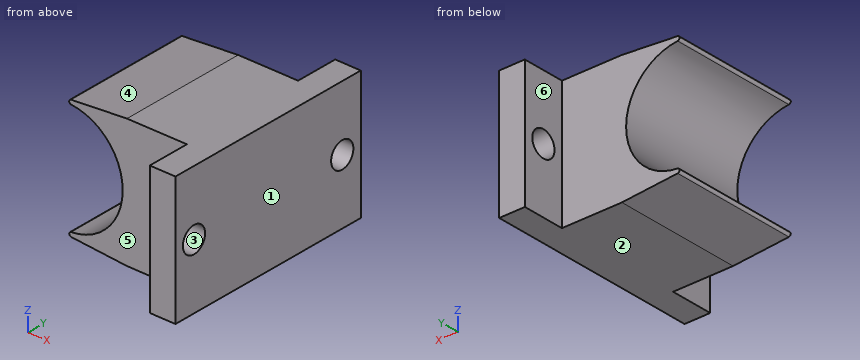
```python
from build123d import *

# Parameters (mm, degrees)
SKETCH003_W     = 5
SKETCH003_H     = 25
SKETCH003_R     = 1.5
PAD001_DEPTH    = 10
SKETCH004_W     = 5
SKETCH004_H     = 5
POCKET002_DEPTH = 7
PAD009_DEPTH    = 5
PAD010_DEPTH    = 5
PAD011_DEPTH    = 15


with BuildPart() as part:
    # Sketch003 (on DatumPlane) → Pad001 (new body)
    with BuildSketch(Plane(origin=(0, 0, 0), x_dir=(0, 0, -1), z_dir=(-1, 0, 0))):
        with Locations((-10, 20)):
            Rectangle(SKETCH003_W, SKETCH003_H)
        with Locations((-10, 30)):
            Circle(SKETCH003_R, mode=Mode.SUBTRACT)
        with Locations((-10, 10)):
            Circle(SKETCH003_R, mode=Mode.SUBTRACT)
    extrude(amount=PAD001_DEPTH)

    # Sketch004 (on Face8 of Pad001) → Pocket002 (cut)
    with BuildSketch(Plane(origin=(-10, 0, 0), x_dir=(0, 0, -1), z_dir=(-1, 0, 0))):
        with Locations((-10, 30)):
            Rectangle(SKETCH004_W, SKETCH004_H)
        with Locations((-10, 10)):
            Rectangle(SKETCH004_W, SKETCH004_H)
    extrude(amount=-POCKET002_DEPTH, mode=Mode.SUBTRACT)

    # Pocket002 Face3 → Pad009 (add)
    with BuildSketch(Plane(origin=(-4.416667, -20, 7.5), x_dir=(0, -1, 0), z_dir=(0, 0, -1))):
        Polygon((-12.5, -4.416667), (12.5, -4.416667), (12.5, -1.416667), (7.5, -1.416667), (7.5, 5.583333), (-7.5, 5.583333), (-7.5, -1.416667), (-12.5, -1.416667), align=None)
    extrude(amount=PAD009_DEPTH)

    # Pad009 Face3 → Pad010 (add)
    with BuildSketch(Plane(origin=(-4.416667, -20, 12.5), x_dir=(0, 1, 0), z_dir=(0, 0, 1))):
        Polygon((-12.5, -4.416667), (12.5, -4.416667), (12.5, -1.416667), (7.5, -1.416667), (7.5, 5.583333), (-7.5, 5.583333), (-7.5, -1.416667), (-12.5, -1.416667), align=None)
    extrude(amount=PAD010_DEPTH)

    # Sketch020 (on Face11 of Pad010) → Pad011 (join)
    with BuildSketch(Plane(origin=(0, -12.5, 0), x_dir=(0, 0, -1), z_dir=(0, 1, 0))):
        with BuildLine():
            ThreePointArc((-16.482143, 16.518519), (-10, 10.5), (-3.517857, 16.518519))
            ThreePointArc((-3.019333, 16.519851), (-3.269212, 16.749999), (-3.517857, 16.518519))
            Line((-2.5, 10), (-3.019333, 16.519851))
            Line((-2.5, 10), (-10, 10))
            Line((-17.5, 10), (-10, 10))
            Line((-17.5, 10), (-16.980667, 16.519851))
            ThreePointArc((-16.482143, 16.518519), (-16.730788, 16.749999), (-16.980667, 16.519851))
        make_face()
    extrude(amount=-PAD011_DEPTH)


solid = part.part
```
Check sheet for the modelled part. Datum: model origin and axes. Units: mm. Face numbers are marked on the shaded views. A direction names the side the tool comes from. Round coordinates to 2 decimals unless told otherwise and drop trailing zeros. Order: outer loops, then holes, each group sorted by start corner. A loop starts at its lowest first (then second) coordinate and runs counter-clockwise, first axis right, second up. Notation, with made-up numbers: (-17, 37.25) - (8, 37.25) arc R8 ccw to (8, 43.25) - close; hole circle Ø3 at (12, 37.25). An arc over 180 degrees is marked (long way). Write item = value, one per line.
Q1. Thickness scan on line 1 along Y through (x, z) = (-1.35, 10); line 2 along Z through (x, y) = (-0.85, -30); line 3 along X through (y, z) = (-11.5, 14.75). Record the ranges inside material, lowest first.
Computed:
line_1 = -32.5 to -31.5, -28.5 to -11.5, -8.5 to -7.5
line_2 = 2.5 to 8.5, 11.5 to 17.5
line_3 = -3 to 0
Q2. Go/stop test with flat-tipped pins: pin 1 (4 mm diameter, centred on x = -13.5, y = -12, fed in from +Z); pin 2 (6 mm diameter, centred on x = -12.5, z = 7, fed in from -Y); pin 3 (1.5 mm diameter, centred on y = -29, z = 8.5, fed in from -X). Record where each tip stops, or that it passes through.
Computed:
pin_1 = 17.38
pin_2 = -27.5
pin_3 = -3
Q3. Section check C-C (y = -10). Record the boundary of the cut face in (x, z), and give its area (3 significant figures).
Computed:
outline = (-3, 2.5) - (0, 2.5) - (0, 8.5) - (-3, 8.5) - close; (-3, 11.5) - (0, 11.5) - (0, 17.5) - (-3, 17.5) - close
area = 36.0 mm^2
Q4. Tool access check on the marked faces 4, 5 and 6. Record the directions out of +Z, -Z, +X, -X, +Y, -Y that give a thin tool (end or side, any length) a straight path to the whole face; none if there is none.
Computed:
face_4 = +Z, -X, +Y, -Y
face_5 = +Z, -Z, -X, -Y
face_6 = +Z, -Z, -X, +Y
Q5. Draft check along Z on the marked faces 1, 2 and 3. Enter one of: pulls with the +Z half, pulls with the -Z half, needs draft (parallel to the pull), parting line crosses it, or undercut.
Computed:
face_1 = needs draft
face_2 = pulls with the -Z half
face_3 = undercut
Q6. Section check A-A (z = 10). Record the boundary of the cut face in (x, y), and give its area (4 significant figures).
Computed:
outline = (-10.5, -27.5) - (-3, -27.5) - (-3, -28.5) - (0, -28.5) - (0, -11.5) - (-3, -11.5) - (-3, -12.5) - (-10.5, -12.5) - close; (-3, -32.5) - (0, -32.5) - (0, -31.5) - (-3, -31.5) - close; (-3, -8.5) - (0, -8.5) - (0, -7.5) - (-3, -7.5) - close
area = 169.5 mm^2
Q7. Section check B-B (x = -15). Record the boundary of the cut face in (y, z), and give its area (3 significant figures).
Computed:
outline = (-27.5, 2.9) - (-12.5, 2.9) - (-12.5, 3.82) - (-27.5, 3.82) - close; (-27.5, 16.18) - (-12.5, 16.18) - (-12.5, 17.1) - (-27.5, 17.1) - close
area = 27.5 mm^2
Q8. Section check D-D (y = -20.75). Record the boundary of the cut face in (x, z).
Computed:
outline = (-16.52, 3.02) - (-10, 2.5) - (0, 2.5) - (0, 17.5) - (-10, 17.5) - (-16.52, 16.98) arc R0.25 ccw to (-16.52, 16.48) arc R6.5 cw to (-16.52, 3.52) arc R0.25 ccw to start
